Part print with two shaded views. Sizes in mm from the minimum x, y, z corner. Round coordinates to 2 decimals unless told otherwise and drop trailing zeros. Loops run counter-clockwise (first coordinate to the right, second up) from the corner with the lowest first, then second, coordinate; pieces in that order, holes last. Notation, with made-up numbers: M 5,26.5 L 16,26.5 A31 cw 16,53.5 Z; hole C -40,-31.75 d2. An arc over 180 degrees is marked long. Use a Markdown table: item, result. Add a question column.
Item 1: Two-plate mould, pull along X, no slides. Class the marked faces 1, 2 and 3: +X half, -X half, draft (parallel to the pull), parting line (faces both ways), or undercut.
Item 2: Saw through at C-C on z = 1.25. Write the cut outline in (x, y), then the cut area to 3 significant figures.
Item 3: Saw through at A-A on y = 17.5. Write the cut outline in (x, z), then the cut area to 3 significant figures.
Item 4: Pin check, flat tips, straight feed: P1, Ø5, axis at y = 30, z = 6.5, coming from the -X side; P2, Ø4, axis at x = 25.5, z = 1, coming from the -Y side; P3, Ø3, axis at y = 9.5, z = 7.5, coming from the +X side; P4, Ø11.5, axis at x = 17.5, y = 17.5, coming from the -Z side. Stop position of each tip, or through.
Item 5: Wall check: L1, parallel to Y at x = 17.5, z = 6.75; L2, parallel to Y at x = 17.5, z = 5.5; L3, parallel to X at y = 23, z = 9.5. Give the ranges that are in metal, low to high. Write a range as from..to.
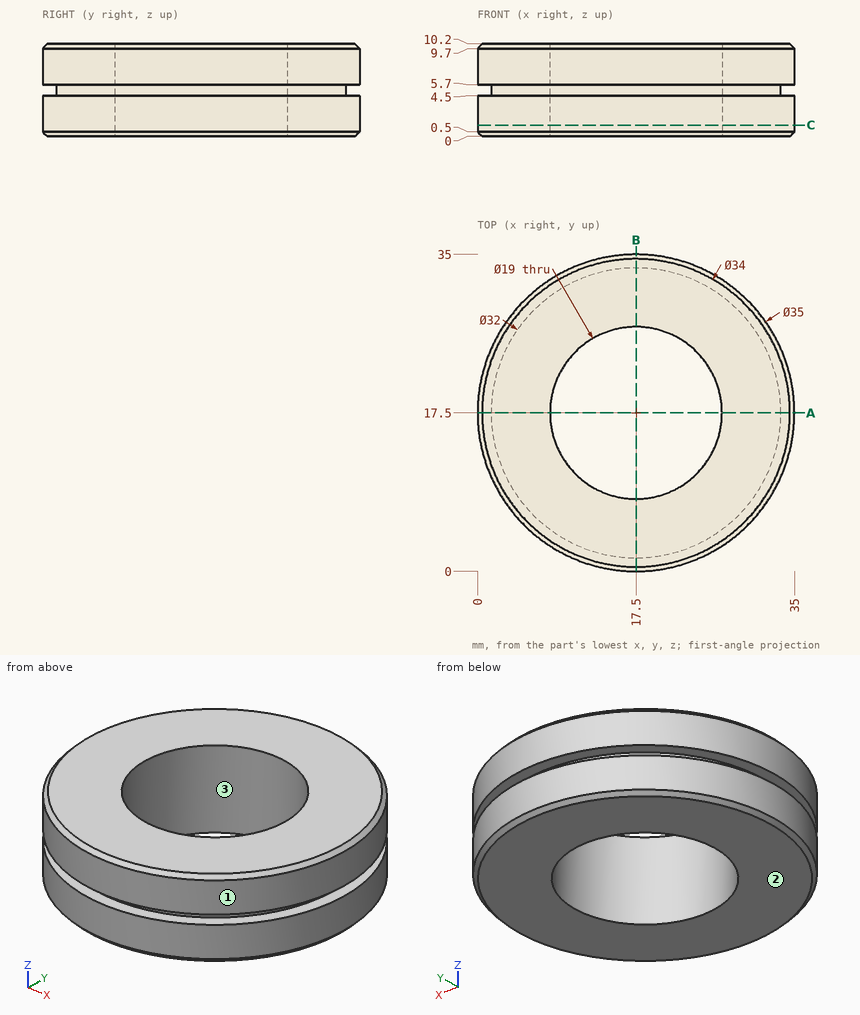
Entries:
| question | item | result |
|---|---|---|
| 1 | face 1 | parting line |
| 1 | face 2 | draft |
| 1 | face 3 | undercut |
| 2 | outline | C 17.5,17.5 d35; hole C 17.5,17.5 d19 |
| 2 | area | 679 mm2 |
| 3 | outline | M 0,0.5 L 0.5,0 L 8,0 L 8,10.2 L 0.5,10.2 L 0,9.7 L 0,5.7 L 1.5,5.7 L 1.5,4.5 L 0,4.5 Z; M 27,0 L 34.5,0 L 35,0.5 L 35,4.5 L 33.5,4.5 L 33.5,5.7 L 35,5.7 L 35,9.7 L 34.5,10.2 L 27,10.2 Z |
| 3 | area | 159 mm2 |
| 4 | P1 | x = 3.14 |
| 4 | P2 | y = 1.06 |
| 4 | P3 | x = 33.75 |
| 4 | P4 | through |
| 5 | L1 | 0..8, 27..35 |
| 5 | L2 | 1.5..8, 27..33.5 |
| 5 | L3 | 0.89..9.75, 25.25..34.11 |
